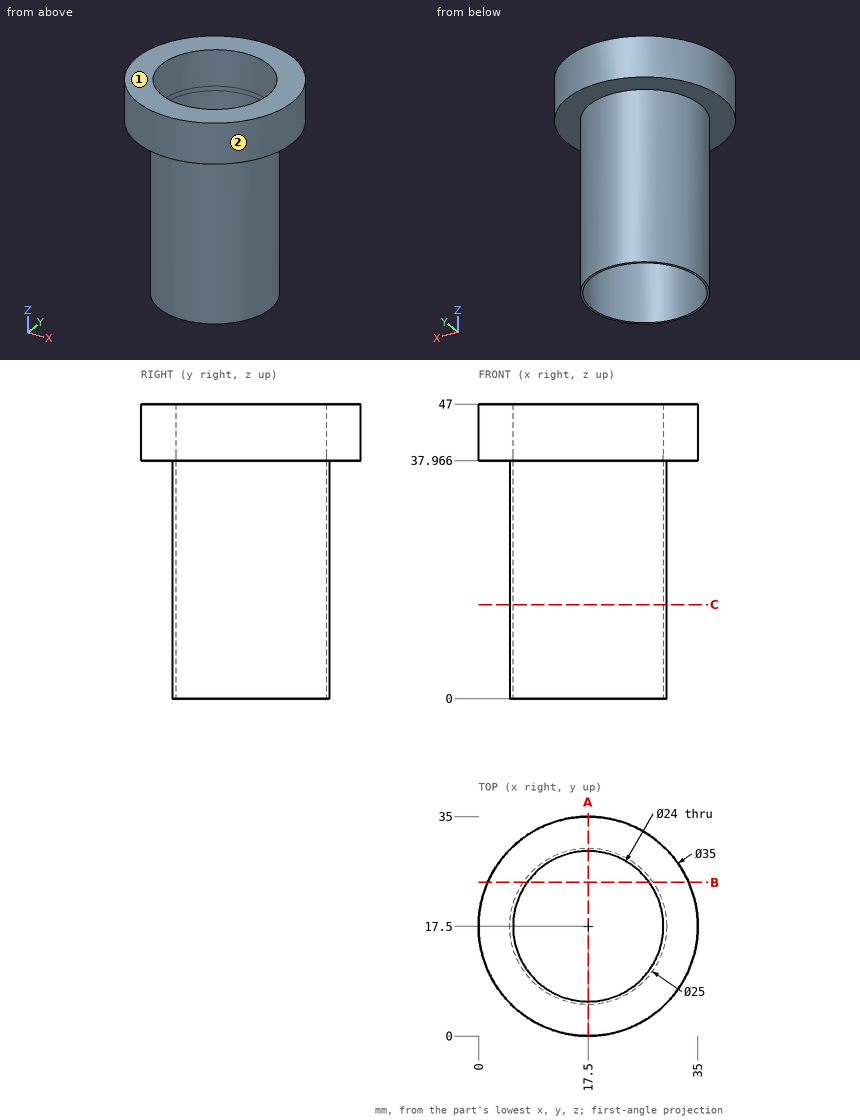
The drawing under review shows one solid part. Ordinate dimensions are in mm from its lowest x, y, z. Round coordinates to 2 decimals unless told otherwise and drop trailing zeros. Loops run counter-clockwise (first coordinate to the right, second up) from the corner with the lowest first, then second, coordinate; pieces in that order, holes last. Notation, with made-up numbers: (38.5, 78.25) - (94.5, 78.25) arc R17 ccw to (94.5, 90.25) - close; hole circle Ø9 at (64, -38.75). An arc over 180 degrees is marked (long way). Use a Markdown table: item, result. Add a question column.
Q1. Add section C-C (z = 15). State the section outline as (x, y) points.
Q2. Add section B-B (y = 24.5). State the section outline as (x, z) points, plus the area to 3 significant figures.
Q3. For probe 1 along Y at (x, z) = (17, 38); probe 2 along Y at (x, z) = (18, 11); probe 3 along X at (y, z) = (17.5, 16), list the stretches that pass through material, from the lowest coordinate up.
Q4. The part is to be moulded in two halves that separate along Y. For the marked faces 1 and 2, say which applies: pulls with the +Y half, pulls with the -Y half, needs draft (parallel to the pull), parting line crosses it, or undercut.
Q5. Insertion check: pin 1 Ø4 at (x, y) = (9.5, 25) entering from +Z; pin 2 Ø4 at (x, z) = (8, 5) entering from +Y; pin 3 Ø14.5 at (x, y) = (17.5, 17.5) entering from +Z; pin 4 Ø2 at (x, z) = (19.5, 25.5) entering from -Y. Each pin has a flat end and moves straight along its axis. Give the tip position at first contact, or say it passes through.
Q6. Add section A-A (x = 17.5). State the section outline as (y, z) points, plus the area to 3 significant figures.
Worked answers:
| question | item | result |
|---|---|---|
| 1 | outline | circle Ø25 at (17.5, 17.5); hole circle Ø24 at (17.5, 17.5) |
| 2 | outline | (1.46, 37.97) - (7.14, 37.97) - (7.14, 0) - (7.75, 0) - (7.75, 47) - (1.46, 47) - close; (27.25, 0) - (27.86, 0) - (27.86, 37.97) - (33.54, 37.97) - (33.54, 47) - (27.25, 47) - close |
| 2 | area | 160 mm² |
| 3 | probe 1 | 0.01 to 5.51, 29.49 to 34.99 |
| 3 | probe 2 | 5.01 to 5.51, 29.49 to 29.99 |
| 3 | probe 3 | 5 to 5.5, 29.5 to 30 |
| 4 | face 1 | needs draft |
| 4 | face 2 | parting line crosses it |
| 5 | pin 1 | z = 47 |
| 5 | pin 2 | y = 27.5 |
| 5 | pin 3 | through |
| 5 | pin 4 | y = 5.04 |
| 6 | outline | (0, 37.97) - (5, 37.97) - (5, 0) - (5.5, 0) - (5.5, 47) - (0, 47) - close; (29.5, 0) - (30, 0) - (30, 37.97) - (35, 37.97) - (35, 47) - (29.5, 47) - close |
| 6 | area | 137 mm² |
